The model under review builds one solid part; all positions refer to its coordinate system, in mm. Face numbers are marked on the shaded views. Give positions to 0.01 mm unless a question says otherwise; leave off trailing zeros. Write each loop counter-clockwise with the first axis right and the second up, starting at its lowest first coordinate (ties: lowest second). Pieces come first, ordered by that corner, then holes. Notation, with made-up numbers: (-25, -5.5) -> (-8, -5.5) arc R16 cw to (-8, 22.5) -> close; hole circle Ø10 at (10, 66.25). An arc over 180 degrees is marked (long way). Use CSV: the item, a comma, the result in double quotes.
```python
from build123d import *

# Parameters (mm, degrees)
SKETCH1_R             = 14.29385
SKETCH1_R_2           = 11.1125
BOSS_EXTRUDE1_DEPTH   = 6.35
CROQUIS1_R            = 2.38125
CORTAR_EXTRUIR1_DEPTH = 50
CROQUIS6_R            = 2.38125
CORTAR_EXTRUIR4_DEPTH = 10
CROQUIS7_R            = 2.38125
CORTAR_EXTRUIR5_DEPTH = 10
CROQUIS9_R            = 5
CORTAR_EXTRUIR6_DEPTH = 3.18


with BuildPart() as part:
    # Sketch1 → Boss-Extrude1 (new body)
    with BuildSketch(Plane.XY):
        with BuildLine():
            Line((0, 70), (310, 45))
            ThreePointArc((310, 45), (355, 0), (310, -45))
            Line((310, -45), (5.171398252, -69.808714643))
            ThreePointArc((5.171398252, -69.808714643), (-69.952162315, -2.587467389), (0, 70))
        make_face()
        Circle(SKETCH1_R, mode=Mode.SUBTRACT)
        with Locations((310, 0)):
            Circle(SKETCH1_R, mode=Mode.SUBTRACT)
        with Locations((162.878542763, 35)):
            Circle(SKETCH1_R_2, mode=Mode.SUBTRACT)
        with BuildLine():
            Line((107.898974887, 49.259511156), (143.314248041, 46.40344074))
            ThreePointArc((143.314248041, 46.40344074), (147.389908855, 43.644764005), (147.127454118, 38.730252238))
            Line((147.127454118, 38.730252238), (129.916226305, 11.754586611))
            ThreePointArc((129.916226305, 11.754586611), (125.651076231, 9.444205574), (121.433006579, 11.839462159))
            Line((121.433006579, 11.839462159), (103.228961238, 41.671198203))
            ThreePointArc((103.228961238, 41.671198203), (103.238833139, 46.896293531), (107.898974887, 49.259511156))
        make_face(mode=Mode.SUBTRACT)
        with BuildLine():
            Line((70.523244027, 6), (102.03004784, 6))
            ThreePointArc((102.03004784, 6), (106.3902351, 8.552804247), (106.298140539, 13.604493178))
            Line((106.298140539, 13.604493178), (96.590354482, 29.513051181))
            ThreePointArc((96.590354482, 29.513051181), (88.437172177, 34.296727565), (79.941746192, 30.151166228))
            Line((79.941746192, 30.151166228), (65.58297828, 10.229432452))
            ThreePointArc((65.58297828, 10.229432452), (67.271539685, 7.201787411), (70.523244027, 6))
        make_face(mode=Mode.SUBTRACT)
        with BuildLine():
            Line((219.623774494, 32.810522613), (206.130928429, 12.417497436))
            ThreePointArc((206.130928429, 12.417497436), (201.919524559, 10.176643248), (197.745901529, 12.48710226))
            Line((197.745901529, 12.48710226), (183.296864227, 35.133505128))
            ThreePointArc((183.296864227, 35.133505128), (183.227765467, 40.400743015), (187.913912204, 42.80669363))
            Line((187.913912204, 42.80669363), (215.855795571, 40.553315939))
            ThreePointArc((215.855795571, 40.553315939), (219.949772588, 37.757395035), (219.623774494, 32.810522613))
        make_face(mode=Mode.SUBTRACT)
        with BuildLine():
            Line((96.590354482, -29.513051181), (106.298140539, -13.604493178))
            ThreePointArc((106.298140539, -13.604493178), (106.3902351, -8.552804247), (102.03004784, -6))
            Line((102.03004784, -6), (70.523244027, -6))
            ThreePointArc((70.523244027, -6), (67.271539685, -7.201787411), (65.58297828, -10.229432452))
            Line((65.58297828, -10.229432452), (79.941746192, -30.151166228))
            ThreePointArc((79.941746192, -30.151166228), (88.437172177, -34.296727565), (96.590354482, -29.513051181))
        make_face(mode=Mode.SUBTRACT)
        with BuildLine():
            Line((187.913912204, -42.80669363), (215.855795571, -40.553315939))
            ThreePointArc((215.855795571, -40.553315939), (219.949772588, -37.757395035), (219.623774494, -32.810522613))
            Line((219.623774494, -32.810522613), (206.130928429, -12.417497436))
            ThreePointArc((206.130928429, -12.417497436), (201.919524559, -10.176643248), (197.745901529, -12.48710226))
            Line((197.745901529, -12.48710226), (183.296864227, -35.133505128))
            ThreePointArc((183.296864227, -35.133505128), (183.227765467, -40.400743015), (187.913912204, -42.80669363))
        make_face(mode=Mode.SUBTRACT)
        with BuildLine():
            Line((121.433006579, -11.839462159), (103.228961238, -41.671198203))
            ThreePointArc((103.228961238, -41.671198203), (103.238833139, -46.896293531), (107.898974887, -49.259511156))
            Line((107.898974887, -49.259511156), (143.314248041, -46.40344074))
            ThreePointArc((143.314248041, -46.40344074), (147.389908855, -43.644764005), (147.127454118, -38.730252238))
            Line((147.127454118, -38.730252238), (129.916226305, -11.754586611))
            ThreePointArc((129.916226305, -11.754586611), (125.651076231, -9.444205574), (121.433006579, -11.839462159))
        make_face(mode=Mode.SUBTRACT)
    extrude(amount=BOSS_EXTRUDE1_DEPTH)

    # Croquis1 → Cortar-Extruir1 (cut)
    with BuildSketch(Plane.XY.offset(6.35)):
        with Locations((98.995555235, -37.090103176)):
            Circle(CROQUIS1_R)
        with Locations((228.877351461, -26.519571404)):
            Circle(CROQUIS1_R)
    extrude(amount=-CORTAR_EXTRUIR1_DEPTH, mode=Mode.SUBTRACT)

    # Croquis6 → Cortar-Extruir4 (cut)
    with BuildSketch(Plane(origin=(0, 0, 0), x_dir=(-1, 0, 0), z_dir=(0, 0, -1))):
        with Locations((-162.878542763, -5)):
            Circle(CROQUIS6_R)
    extrude(amount=-CORTAR_EXTRUIR4_DEPTH, mode=Mode.SUBTRACT)

    # Croquis7 → Cortar-Extruir5 (cut)
    with BuildSketch(Plane(origin=(0, 0, 0), x_dir=(-1, 0, 0), z_dir=(0, 0, -1))):
        with Locations((-65.84135797, 50.868973694)):
            Circle(CROQUIS7_R)
        with Locations((-262.871569638, 39.210126075)):
            Circle(CROQUIS7_R)
    extrude(amount=-CORTAR_EXTRUIR5_DEPTH, mode=Mode.SUBTRACT)

    # Croquis9 → Cortar-Extruir6 (cut)
    with BuildSketch(Plane.XY.offset(6.35)):
        with Locations((65.84135797, 50.868973694)):
            Circle(CROQUIS9_R)
        with Locations((162.878542763, -5)):
            Circle(CROQUIS9_R)
        with Locations((98.995555235, -37.090103176)):
            Circle(CROQUIS9_R)
        with Locations((228.877351461, -26.519571404)):
            Circle(CROQUIS9_R)
        with Locations((262.871569638, 39.210126075)):
            Circle(CROQUIS9_R)
    extrude(amount=-CORTAR_EXTRUIR6_DEPTH, mode=Mode.SUBTRACT)


solid = part.part
```
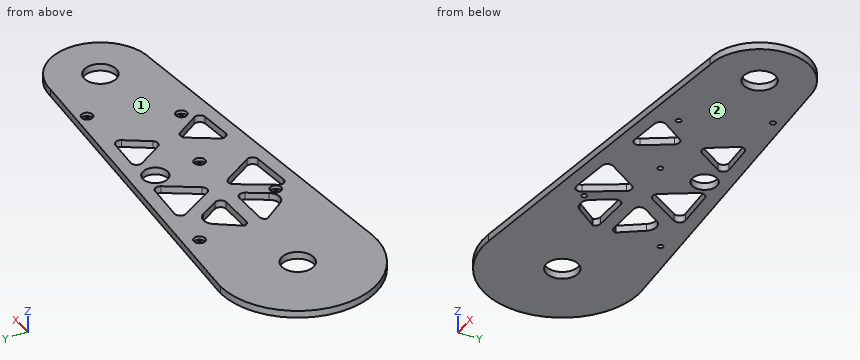
Q1. The part is to be moulded in two halves that separate along Z. For the marked faces 1 and 2, say which applies: pulls with the +Z half, pulls with the -Z half, needs draft (parallel to the pull), parting line crosses it, or undercut.
Derived:
face 1,"pulls with the +Z half"
face 2,"pulls with the -Z half"
Q2. Consider section B-B (y = -57). Write out the cut boundary in (x, z), then the cut area to 3 significant figures.
Derived:
outline,"(-40.63, 0) -> (162.55, 0) -> (162.55, 6.35) -> (-40.63, 6.35) -> close"
area,"1,290 mm2"
Q3. Consider section A-A (z = 1.5). State how many separate pieces and enclosed holes the cut face has, then the cut area to 3 significant figures.
Derived:
separate pieces,"1"
enclosed holes,"14"
area,"39,500 mm2"
Q4. To check wall thickness, follow probe 1 along X at (y, z) = (-23.5, 1.5); probe 2 along X at (y, z) = (-40, 5.75); probe 3 along Y at (x, z) = (131.5, 4.5). State the ranges of each line that lie inside material, in increasing order.
Derived:
probe 1,"x = -65.94 to 75.15, 100.26 to 114.32, 137.41 to 190.72, 213.46 to 348.38"
probe 2,"x = -57.45 to 94.93, 103.06 to 104.25, 147.71 to 183.01, 217.77 to 330.62"
probe 3,"y = -59.53 to -47.36, -14.24 to 14.24, 47.36 to 59.4"
Q5. Insertion check: pin 1 (5 mm diameter, centred on x = 97.5, y = -35.5, fed in from +Z); pin 2 (1.5 mm diameter, centred on x = 197.5, z = 3.5, fed in from +Y); pin 3 (1.5 mm diameter, centred on x = 290.5, y = -43.5, fed in from -Z); pin 4 (1.9 mm diameter, centred on x = 93.5, z = 2, fed in from +Y). Each pin has a flat end and moves straight along its axis. Give the tip position at first contact, or say it passes through.
Derived:
pin 1,"stops at z = 3.17"
pin 2,"stops at y = 54.13"
pin 3,"stops at z = 0"
pin 4,"stops at y = 62.54"
